CAD build for the part. Positions are in the model's coordinates, mm. A direction names the side the tool comes from. Give positions to 0.01 mm unless a question says otherwise; leave off trailing zeros. Write each loop counter-clockwise with the first axis right and the second up, starting at its lowest first coordinate (ties: lowest second). Pieces come first, ordered by that corner, then holes. Notation, with made-up numbers: (68.5, 15.25) -> (96.5, 15.25) arc R31 cw to (96.5, 48.25) -> close; hole circle Ø4 at (-11, -28.5). An arc over 180 degrees is marked (long way). Answer as a JSON object with one key per item and string values.
```python
from build123d import *

# Parameters (mm, degrees)
BOSS_EXTRUDE1_DEPTH = 10
SKETCH2_R           = 4
CUT_EXTRUDE1_DEPTH  = 10
BOSS_EXTRUDE2_DEPTH = 5
BOSS_EXTRUDE3_DEPTH = 5
FILLET1_R           = 1


with BuildPart() as part:
    # Sketch1 → Boss-Extrude1 (new body)
    with BuildSketch(Plane.XY):
        with BuildLine():
            Line((-10, -20), (10, -20))
            Line((10, -20), (10, 10))
            ThreePointArc((10, 10), (0, 20), (-10, 10))
            Line((-10, 10), (-10, -20))
        make_face()
    extrude(amount=BOSS_EXTRUDE1_DEPTH)

    # Sketch2 → Cut-Extrude1 (cut)
    with BuildSketch(Plane(origin=(0, 0, 0), x_dir=(-1, 0, 0), z_dir=(0, 0, -1))):
        with Locations((0, 10)):
            Circle(SKETCH2_R)
    extrude(amount=-CUT_EXTRUDE1_DEPTH, mode=Mode.SUBTRACT)

    # Sketch3 → Boss-Extrude2 (add)
    with BuildSketch(Plane.XZ.offset(20)):
        with BuildLine():
            Line((-8, 7), (8, 7))
            ThreePointArc((8, 7), (10, 5), (8, 3))
            Line((8, 3), (-8, 3))
            ThreePointArc((-8, 3), (-10, 5), (-8, 7))
        make_face()
    extrude(amount=BOSS_EXTRUDE2_DEPTH)

    # Sketch4 → Boss-Extrude3 (add)
    with BuildSketch(Plane.XZ.offset(20)):
        Polygon((-1.75, 8), (1.75, 8), (3, 8), (3, 6.75), (3, 3.25), (3, 2), (1.75, 2), (-1.75, 2), (-3, 2), (-3, 3.25), (-3, 6.75), (-3, 8), align=None)
    extrude(amount=BOSS_EXTRUDE3_DEPTH)

    # Fillet1
    fillet1_edges = [part.edges().sort_by_distance(p)[0] for p in [
        (3, -22.5, 7),
        (3, -22.5, 3),
        (-3, -22.5, 3),
        (-3, -22.5, 7),
    ]]
    fillet(fillet1_edges, radius=FILLET1_R - 0.0001)  # a hair under: the kernel refuses the full size


solid = part.part
```
1) 3-axis set-ups, long thin cutter, end or side, ignore diameter. For faces 1 (the flat face through (0, -22, 2)), 2 (the cylindrical face through (-3.285, -22.465, 7.301)), 3 (the cylindrical face through (-10, -22, 5)), 4 (the cylindrical face through (3.285, -22.535, 7.301)): which of +Z, -Z, +X, -X, +Y, -Y reach the whole face in a straight line?
Model answer:
{"face 1": "-Z, +X, -X, -Y", "face 2": "+Z, -X, -Y", "face 3": "-X, -Y", "face 4": "+Z, +X, -Y"}
2) Pin check, flat tips, straight feed: pin 1 (4 mm diameter, centred on x = -6, z = 2.5, fed in from +Y); pin 2 (4 mm diameter, centred on x = 0.5, y = -22.5, fed in from +Z); pin 3 (4.5 mm diameter, centred on x = 5.5, y = -23, fed in from -Z). Stop position of each tip, or through.
Model answer:
{"pin 1": "stops at y = 19.17", "pin 2": "stops at z = 8", "pin 3": "stops at z = 2.66"}
3) Wall check: probe 1 along Y at (x, z) = (0, 2.5); probe 2 along Y at (x, z) = (3, 5.25); probe 3 along X at (y, z) = (9.5, 3). Give the ranges that are in metal, low to high.
Model answer:
{"probe 1": "y = -25 to 6, 14 to 20", "probe 2": "y = -25 to 7.35, 12.65 to 19.54", "probe 3": "x = -10 to -3.97, 3.97 to 10"}
4) Slice it at A-A (x = -3.5). List the corners of the cut face in (y, z).
Model answer:
{"outline": "(-25, 2.87) -> (-20, 2.87) -> (-20, 0) -> (8.06, 0) -> (8.06, 10) -> (-20, 10) -> (-20, 7.13) -> (-25, 7.13) -> close; (11.94, 0) -> (19.37, 0) -> (19.37, 10) -> (11.94, 10) -> close"}
5) Slice it at B-B (z = 1). List the corners of the cut face in (x, y), then the cut area to 3 significant figures.
Model answer:
{"outline": "(-10, -20) -> (10, -20) -> (10, 10) arc R10 ccw to (-10, 10) -> close; hole circle Ø8 at (0, 10)", "area": "707 mm2"}
6) Slice it at C-C (y = 13). List the corners of the cut face in (x, z).
Model answer:
{"outline": "(-9.54, 0) -> (-2.65, 0) -> (-2.65, 10) -> (-9.54, 10) -> close; (2.65, 0) -> (9.54, 0) -> (9.54, 10) -> (2.65, 10) -> close"}
